```python
from build123d import *

# Parameters (mm, degrees)
F0_W     = 152.4
F0_H     = 152.4
F1_DEPTH = 9.525
F2_W     = 133.35
F2_H     = 133.35
F3_DEPTH = 9.525
F5_D     = 12.7


with BuildPart() as f1:
    # F0 (on Top) → F1 (new body)
    with BuildSketch(Plane.XY):
        Rectangle(F0_W, F0_H)
    extrude(amount=F1_DEPTH)

    # F2 (on face) → F3 (join)
    with BuildSketch(Plane(origin=(0, 0, 0), x_dir=(1, 0, 0), z_dir=(0, 0, -1))):
        Rectangle(F2_W, F2_H)
    extrude(amount=F3_DEPTH)

    # F5 (through all)
    with Locations(Plane.XY.offset(9.525)):
        with Locations((0, 0)):
            Hole(F5_D / 2)


solid = f1.part
```
Source: CAD feature listing. Evaluate the final solid. Frame: model axes, mm. A direction names the side the tool comes from. Give positions to 0.01 mm unless a question says otherwise; leave off trailing zeros. Write each loop counter-clockwise with the first axis right and the second up, starting at its lowest first coordinate (ties: lowest second). Pieces come first, ordered by that corner, then holes.
1. Pull-direction query (X, two-part tool) for faces 1 (the face through (-76.2, -1, 5)), 2 (the face through (-1, -66.675, -5)), 3 (the face through (1.38, -6.2, -0.13)); classes: +X half, -X half, draft (parallel to the pull), parting line (faces both ways), or undercut.
2. Material intervals for line 1 along Y through (x, z) = (0, -0.75) (3 decimals); line 2 along Z through (x, y) = (16.5, -67.5) (3 decimals); line 3 along Y through (x, z) = (-61.5, -6.5) (3 decimals), sorted ascending.
3. First-contact query: pin 1 (3 mm diameter, centred on y = -10.5, z = -3.5, fed in from +X) (3 decimals); pin 2 (5 mm diameter, centred on x = 6, z = -6, fed in from +Y) (3 decimals); pin 3 (1 mm diameter, centred on x = -52, z = -6, fed in from -Y) (3 decimals). Flat tips, straight axial feed; report the tip coordinate or a pass-through.
4. Access query for faces 4 (the face through (66.675, 1, -5)), 5 (the face through (-66.675, 1, -5)), 6 (the face through (-1, 66.675, -5)). Directions: +Z, -Z, +X, -X, +Y, -Y. A direction counts if a zero-diameter tool reaches every point of the face in a straight line with its end or side. Return the directions, or none.
5. Section query A-A (y = 0). Return the cut outline in (x, z) (3 decimals).
6. Section query C-C (x = -38). Return the cut outline in (y, z) (3 decimals).
Output values:
1. face 1: -X half
1. face 2: draft
1. face 3: undercut
2. line 1: y = -66.675 to -6.35, 6.35 to 66.675
2. line 2: z = 0 to 9.525
2. line 3: y = -66.675 to 66.675
3. pin 1: stops at x = 66.675
3. pin 2: stops at y = 66.675
3. pin 3: stops at y = -66.675
4. face 4: -Z, +X, +Y, -Y
4. face 5: -Z, -X, +Y, -Y
4. face 6: -Z, +X, -X, +Y
5. outline: (-76.2, 0) - (-66.675, 0) - (-66.675, -9.525) - (-6.35, -9.525) - (-6.35, 9.525) - (-76.2, 9.525) - close; (6.35, -9.525) - (66.675, -9.525) - (66.675, 0) - (76.2, 0) - (76.2, 9.525) - (6.35, 9.525) - close
6. outline: (-76.2, 0) - (-66.675, 0) - (-66.675, -9.525) - (66.675, -9.525) - (66.675, 0) - (76.2, 0) - (76.2, 9.525) - (-76.2, 9.525) - close
